Job drawing, mm, ordinate dimensions from the low corner. One solid piece. Give positions to 0.01 mm unless a question says otherwise; leave off trailing zeros. Loops run counter-clockwise (first coordinate to the right, second up) from the corner with the lowest first, then second, coordinate; pieces in that order, holes last. Notation, with made-up numbers: (60, 79) - (107, 79) arc R18 cw to (107, 88) - close; hole circle Ø9 at (78, 43.5). An arc over 180 degrees is marked (long way). Answer as CSV lines item,"result". Start each with the question number.
Item 1: Saw through at D-D on y = 0.7. Give the cut face in (x, z), plus the area to 3 significant figures.
Item 2: Saw through at C-C on z = 8. Give the cut face in (x, y), plus the area to 3 significant figures.
Item 3: Pin check, flat tips, straight feed: pin 1 (1.8 mm diameter, centred on x = 2.5, y = 2.5, fed in from +Z); pin 2 (1 mm diameter, centred on y = 4, z = 21.5, fed in from +X). Stop position of each tip, or through.
Item 4: Drill centre lines: L1, parallel to Y at x = 2.5, z = 38.25; L2, parallel to X at y = 2.9, z = 18.5; L3, parallel to X at y = 1.95, z = 32.5. Where is each one in solid material? Low to high. Write a range as from..to.
Item 5: Saw through at A-A on x = 2.5. Give the cut face in (y, z).
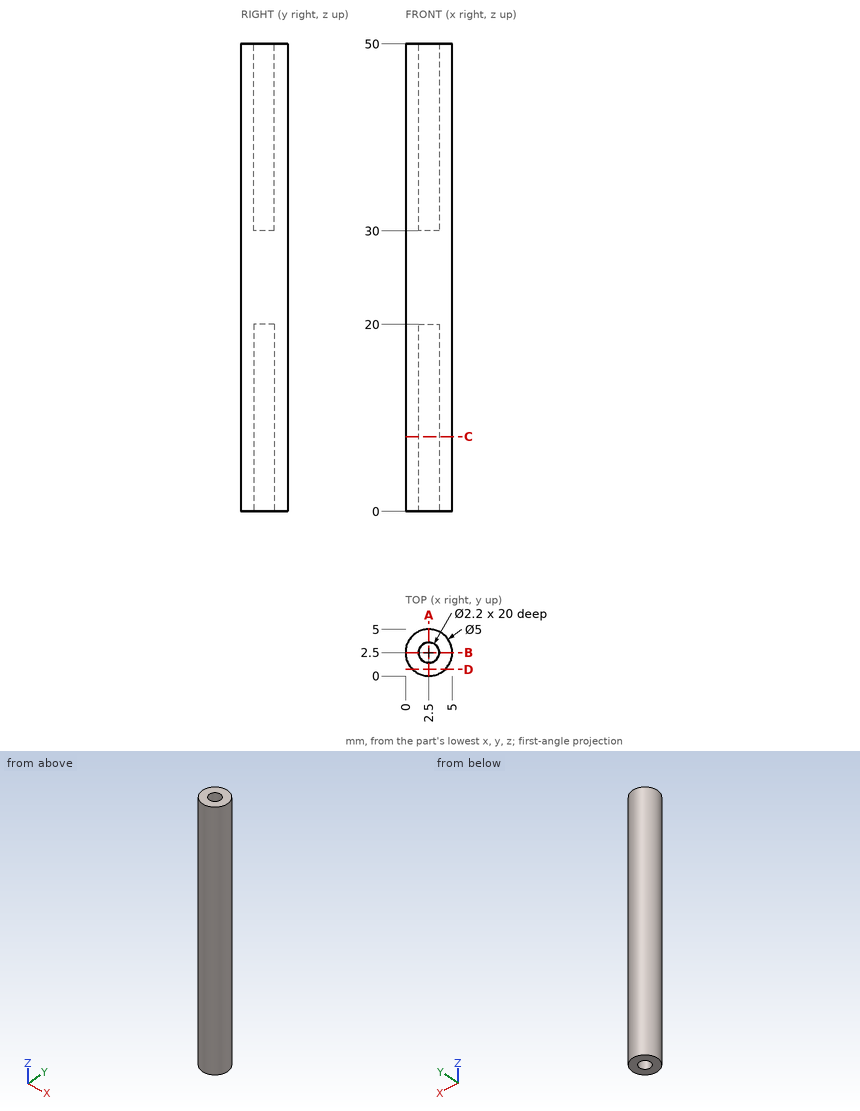
Responses:
1,outline,"(0.77, 0) - (4.23, 0) - (4.23, 50) - (0.77, 50) - close"
1,area,"173 mm2"
2,outline,"circle Ø5 at (2.5, 2.5); hole circle Ø2.2 at (2.5, 2.5)"
2,area,"15.8 mm2"
3,pin 1,"z = 30"
3,pin 2,"x = 4.79"
4,L1,"0..1.4, 3.6..5"
4,L2,"0.03..1.48, 3.52..4.97"
4,L3,"0.06..1.55, 3.45..4.94"
5,outline,"(0, 0) - (1.4, 0) - (1.4, 20) - (3.6, 20) - (3.6, 0) - (5, 0) - (5, 50) - (3.6, 50) - (3.6, 30) - (1.4, 30) - (1.4, 50) - (0, 50) - close"
